The listing builds one solid part. Answer for the finished solid, in the listing's coordinates (mm). A direction names the side the tool comes from. Round coordinates to 2 decimals unless told otherwise and drop trailing zeros. Order: outer loops, then holes, each group sorted by start corner. A loop starts at its lowest first (then second) coordinate and runs counter-clockwise, first axis right, second up. Notation, with made-up numbers: (-4, 84.5) -> (5, 84.5) arc R16 ccw to (5, 114.5) -> close; hole circle Ø6 at (11, 20.25). An arc over 180 degrees is marked (long way). Return JSON: item names as keys, results as strings. Group by question number.
(1) Consider line 1 (Y direction, x = 0, z = 2.5) (3 decimals); line 2 (Y direction, x = 26.5, z = 4.5); line 3 (Y direction, x = 2.5, z = 3.75). Determine where each line is inside the solid, lowest interval first. Write a range as [from, to].
(2) The part is cut by section A-A (x = 0). Determine the outline of the cut face in (y, z) (3 decimals).
(3) Which of the six approach directions +Z, -Z, +X, -X, +Y, -Y give full straight-line access (tool end or side, diameter ignored) to faces 5 (the face through (-8.346, -25.688, 3.131)), 6 (the face through (11.5, 24.44, 3.13)), 7 (the face through (-22.97, 10.84, 3.13)), 8 (the face through (-27, 0, 3))?
(4) Each of these flat-tipped pins is pushed along its axis until it touches: pin 1 (1 mm diameter, centred on x = -7, z = 1, fed in from +Y); pin 2 (2.5 mm diameter, centred on x = 26.5, z = 3.5, fed in from -Y); pin 3 (2 mm diameter, centred on y = -10, z = 3, fed in from -X). Where does it stop, or does it pass through?
(5) Determine the mould class of faces 1 (the face through (1.693, -26.912, 3.131)), 2 (the face through (0.025, 28.575, 3.131)), 3 (the face through (-25.072, -9.927, 3.131)), 4 (the face through (21.851, 15.876, 3.131)) for opening direction X: +X half, -X half, draft (parallel to the pull), parting line (faces both ways), or undercut.
from build123d import *

# Parameters (mm, degrees)
F0_R     = 3.175
F1_DEPTH = 6.35


with BuildPart() as f1:
    # F0 (on Top) → F1 (new body)
    with BuildSketch(Plane.XY):
        with BuildLine():
            Line((-4.759485, 24.950096), (-5.354421, 28.068858))
            ThreePointArc((-5.354421, 28.068858), (-7.106314, 27.677264), (-8.830161, 27.17644))
            Line((-8.830161, 27.17644), (-7.849032, 24.156836))
            ThreePointArc((-7.849032, 24.156836), (-9.350364, 23.616323), (-10.814794, 22.982607))
            Line((-10.814794, 22.982607), (-12.166643, 25.855433))
            ThreePointArc((-12.166643, 25.855433), (-13.766111, 25.040463), (-15.311251, 24.12667))
            Line((-15.311251, 24.12667), (-13.610001, 21.445929))
            ThreePointArc((-13.610001, 21.445929), (-14.929745, 20.549032), (-16.190569, 19.571036))
            Line((-16.190569, 19.571036), (-18.214391, 22.017416))
            ThreePointArc((-18.214391, 22.017416), (-19.560934, 20.830279), (-20.830279, 19.560934))
            Line((-20.830279, 19.560934), (-18.515803, 17.387496))
            ThreePointArc((-18.515803, 17.387496), (-19.571036, 16.190569), (-20.549032, 14.929745))
            Line((-20.549032, 14.929745), (-23.117661, 16.795964))
            ThreePointArc((-23.117661, 16.795964), (-24.12667, 15.311251), (-25.040463, 13.766111))
            Line((-25.040463, 13.766111), (-22.25819, 12.236543))
            ThreePointArc((-22.25819, 12.236543), (-22.982607, 10.814794), (-23.616323, 9.350364))
            Line((-23.616323, 9.350364), (-26.568363, 10.519159))
            ThreePointArc((-26.568363, 10.519159), (-27.17644, 8.830161), (-27.677264, 7.106314))
            Line((-27.677264, 7.106314), (-24.602012, 6.316723))
            ThreePointArc((-24.602012, 6.316723), (-24.950096, 4.759485), (-25.199713, 3.183464))
            Line((-25.199713, 3.183464), (-28.349678, 3.581397))
            ThreePointArc((-28.349678, 3.581397), (-28.518614, 1.794239), (-28.575, 0))
            Line((-28.575, 0), (-25.4, 0))
            ThreePointArc((-25.4, 0), (-25.349879, -1.594879), (-25.199713, -3.183464))
            Line((-25.199713, -3.183464), (-28.349678, -3.581397))
            ThreePointArc((-28.349678, -3.581397), (-28.068858, -5.354421), (-27.677264, -7.106314))
            Line((-27.677264, -7.106314), (-24.602012, -6.316723))
            ThreePointArc((-24.602012, -6.316723), (-24.156836, -7.849032), (-23.616323, -9.350364))
            Line((-23.616323, -9.350364), (-26.568363, -10.519159))
            ThreePointArc((-26.568363, -10.519159), (-25.855433, -12.166643), (-25.040463, -13.766111))
            Line((-25.040463, -13.766111), (-22.25819, -12.236543))
            ThreePointArc((-22.25819, -12.236543), (-21.445929, -13.610001), (-20.549032, -14.929745))
            Line((-20.549032, -14.929745), (-23.117661, -16.795964))
            ThreePointArc((-23.117661, -16.795964), (-22.017416, -18.214391), (-20.830279, -19.560934))
            Line((-20.830279, -19.560934), (-18.515803, -17.387496))
            ThreePointArc((-18.515803, -17.387496), (-17.387496, -18.515803), (-16.190569, -19.571036))
            Line((-16.190569, -19.571036), (-18.214391, -22.017416))
            ThreePointArc((-18.214391, -22.017416), (-16.795964, -23.117661), (-15.311251, -24.12667))
            Line((-15.311251, -24.12667), (-13.610001, -21.445929))
            ThreePointArc((-13.610001, -21.445929), (-12.236543, -22.25819), (-10.814794, -22.982607))
            Line((-10.814794, -22.982607), (-12.166643, -25.855433))
            ThreePointArc((-12.166643, -25.855433), (-10.519159, -26.568363), (-8.830161, -27.17644))
            Line((-8.830161, -27.17644), (-7.849032, -24.156836))
            ThreePointArc((-7.849032, -24.156836), (-6.316723, -24.602012), (-4.759485, -24.950096))
            Line((-4.759485, -24.950096), (-5.354421, -28.068858))
            ThreePointArc((-5.354421, -28.068858), (-3.581397, -28.349678), (-1.794239, -28.518614))
            Line((-1.794239, -28.518614), (-1.594879, -25.349879))
            ThreePointArc((-1.594879, -25.349879), (0, -25.4), (1.594879, -25.349879))
            Line((1.594879, -25.349879), (1.794239, -28.518614))
            ThreePointArc((1.794239, -28.518614), (3.581397, -28.349678), (5.354421, -28.068858))
            Line((5.354421, -28.068858), (4.759485, -24.950096))
            ThreePointArc((4.759485, -24.950096), (6.316723, -24.602012), (7.849032, -24.156836))
            Line((7.849032, -24.156836), (8.830161, -27.17644))
            ThreePointArc((8.830161, -27.17644), (10.519159, -26.568363), (12.166643, -25.855433))
            Line((12.166643, -25.855433), (10.814794, -22.982607))
            ThreePointArc((10.814794, -22.982607), (12.236543, -22.25819), (13.610001, -21.445929))
            Line((13.610001, -21.445929), (15.311251, -24.12667))
            ThreePointArc((15.311251, -24.12667), (16.795964, -23.117661), (18.214391, -22.017416))
            Line((18.214391, -22.017416), (16.190569, -19.571036))
            ThreePointArc((16.190569, -19.571036), (17.387496, -18.515803), (18.515803, -17.387496))
            Line((18.515803, -17.387496), (20.830279, -19.560934))
            ThreePointArc((20.830279, -19.560934), (22.017416, -18.214391), (23.117661, -16.795964))
            Line((23.117661, -16.795964), (20.549032, -14.929745))
            ThreePointArc((20.549032, -14.929745), (21.445929, -13.610001), (22.25819, -12.236543))
            Line((22.25819, -12.236543), (25.040463, -13.766111))
            ThreePointArc((25.040463, -13.766111), (25.855433, -12.166643), (26.568363, -10.519159))
            Line((26.568363, -10.519159), (23.616323, -9.350364))
            ThreePointArc((23.616323, -9.350364), (24.156836, -7.849032), (24.602012, -6.316723))
            Line((24.602012, -6.316723), (27.677264, -7.106314))
            ThreePointArc((27.677264, -7.106314), (28.068858, -5.354421), (28.349678, -3.581397))
            Line((28.349678, -3.581397), (25.199713, -3.183464))
            ThreePointArc((25.199713, -3.183464), (25.349879, -1.594879), (25.4, 0))
            Line((25.4, 0), (28.575, 0))
            ThreePointArc((28.575, 0), (28.518614, 1.794239), (28.349678, 3.581397))
            Line((28.349678, 3.581397), (25.199713, 3.183464))
            ThreePointArc((25.199713, 3.183464), (24.950096, 4.759485), (24.602012, 6.316723))
            Line((24.602012, 6.316723), (27.677264, 7.106314))
            ThreePointArc((27.677264, 7.106314), (27.17644, 8.830161), (26.568363, 10.519159))
            Line((26.568363, 10.519159), (23.616323, 9.350364))
            ThreePointArc((23.616323, 9.350364), (22.982607, 10.814794), (22.25819, 12.236543))
            Line((22.25819, 12.236543), (25.040463, 13.766111))
            ThreePointArc((25.040463, 13.766111), (24.12667, 15.311251), (23.117661, 16.795964))
            Line((23.117661, 16.795964), (20.549032, 14.929745))
            ThreePointArc((20.549032, 14.929745), (19.571036, 16.190569), (18.515803, 17.387496))
            Line((18.515803, 17.387496), (20.830279, 19.560934))
            ThreePointArc((20.830279, 19.560934), (19.560934, 20.830279), (18.214391, 22.017416))
            Line((18.214391, 22.017416), (16.190569, 19.571036))
            ThreePointArc((16.190569, 19.571036), (14.929745, 20.549032), (13.610001, 21.445929))
            Line((13.610001, 21.445929), (15.311251, 24.12667))
            ThreePointArc((15.311251, 24.12667), (13.766111, 25.040463), (12.166643, 25.855433))
            Line((12.166643, 25.855433), (10.814794, 22.982607))
            ThreePointArc((10.814794, 22.982607), (9.350364, 23.616323), (7.849032, 24.156836))
            Line((7.849032, 24.156836), (8.830161, 27.17644))
            ThreePointArc((8.830161, 27.17644), (7.106314, 27.677264), (5.354421, 28.068858))
            Line((5.354421, 28.068858), (4.759485, 24.950096))
            ThreePointArc((4.759485, 24.950096), (3.183464, 25.199713), (1.594879, 25.349879))
            Line((1.594879, 25.349879), (1.794239, 28.518614))
            ThreePointArc((1.794239, 28.518614), (0, 28.575), (-1.794239, 28.518614))
            Line((-1.794239, 28.518614), (-1.594879, 25.349879))
            ThreePointArc((-1.594879, 25.349879), (-3.183464, 25.199713), (-4.759485, 24.950096))
        make_face()
        Circle(F0_R, mode=Mode.SUBTRACT)
    extrude(amount=F1_DEPTH)


solid = f1.part
Answer below:
{
 "1": {"line 1": "y = [-25.4, -3.175], [3.175, 28.575]", "line 2": "y = [-10.69, -10.49], [-6.8, -3.35], [0, 3.35], [6.8, 10.49]", "line 3": "y = [-28.47, -1.96], [1.96, 25.28]"},
 "2": {"outline": "(-25.4, 0) -> (-3.175, 0) -> (-3.175, 6.35) -> (-25.4, 6.35) -> close; (3.175, 0) -> (28.575, 0) -> (28.575, 6.35) -> (3.175, 6.35) -> close"},
 "3": {"face 5": "+Z, -Z, -Y", "face 6": "+Z, -Z, +Y", "face 7": "+Z, -Z", "face 8": "+Z, -Z, -X"},
 "4": {"pin 1": "stops at y = 27.83", "pin 2": "stops at y = -13.38", "pin 3": "stops at x = -26.57"},
 "5": {"face 1": "undercut", "face 2": "parting line", "face 3": "-X half", "face 4": "undercut"}
}
